Part print with two shaded views. Sizes in mm from the minimum x, y, z corner. A direction names the side the tool comes from. Round coordinates to 2 decimals unless told otherwise and drop trailing zeros. Order: outer loops, then holes, each group sorted by start corner. A loop starts at its lowest first (then second) coordinate and runs counter-clockwise, first axis right, second up. Notation, with made-up numbers: (60.5, -10) - (85.5, -10) arc R14 cw to (85.5, 5) - close; hole circle Ø1 at (-2, -1.75). An arc over 180 degrees is marked (long way). Use one line per item in the form item = value.
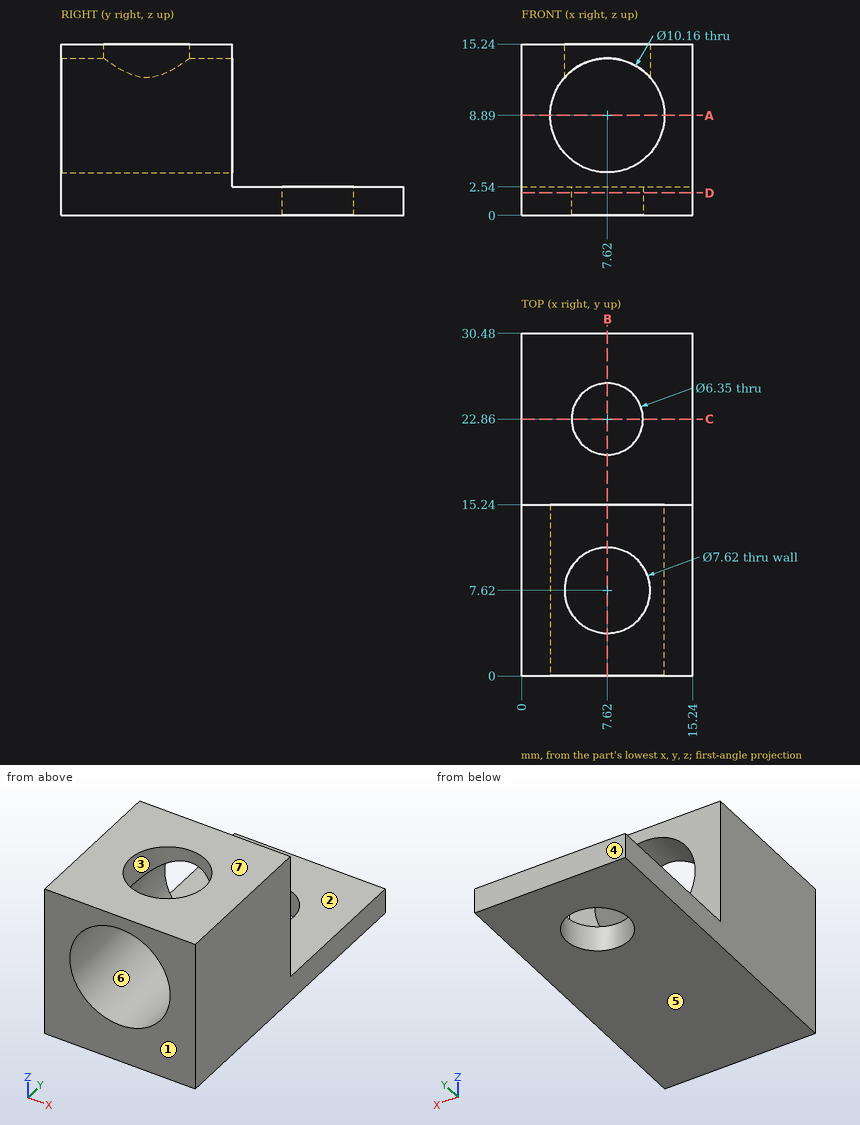
(1) Pull direction Z, two halves, no side cores. Call the marked faces 4, 5, 6 and 7: released by +Z, released by -Z, zero draft, split by the parting line, or undercut.
Report:
face_4 = zero draft
face_5 = released by -Z
face_6 = undercut
face_7 = released by +Z
(2) Slice it at A-A on z = 8.89. Give the cut face in (x, y), then the cut area to 3 significant figures.
Report:
outline = (0, 0) - (2.54, 0) - (2.54, 15.24) - (0, 15.24) - close; (12.7, 0) - (15.24, 0) - (15.24, 15.24) - (12.7, 15.24) - close
area = 77.4 mm2
(3) Slice it at D-D on z = 2. Give the cut face in (x, y) (3 decimals).
Report:
outline = (0, 0) - (15.24, 0) - (15.24, 30.48) - (0, 30.48) - close; hole circle Ø6.35 at (7.62, 22.86)
(4) Probe probe 1 along Y at (x, z) = (7.62, 14); probe 2 along Y at (x, z) = (7.62, 1.05) (3 decimals); probe 3 along Y at (x, z) = (3, 3.75). List the from-to ranges inside material, lowest first. Write a range as [from, to].
Report:
probe_1 = [0, 3.81], [11.43, 15.24]
probe_2 = [0, 19.685], [26.035, 30.48]
probe_3 = [0, 15.24]
(5) Tool access for the marked faces 1, 2 and 3: list every direction of +Z, -Z, +X, -X, +Y, -Y with a clear straight run to the whole face (end or side of a thin tool).
Report:
face_1 = +Z, -Z, +X, -X, -Y
face_2 = +Z, +X, -X, +Y
face_3 = +Z
(6) Slice it at B-B on x = 7.62. Give the cut face in (y, z) (3 decimals), then the cut area to 3 significant figures.
Report:
outline = (0, 0) - (19.685, 0) - (19.685, 2.54) - (15.24, 2.54) - (15.24, 3.81) - (0, 3.81) - close; (0, 13.97) - (3.81, 13.97) - (3.81, 15.24) - (0, 15.24) - close; (11.43, 13.97) - (15.24, 13.97) - (15.24, 15.24) - (11.43, 15.24) - close; (26.035, 0) - (30.48, 0) - (30.48, 2.54) - (26.035, 2.54) - close
area = 90.3 mm2
(7) Pin check, flat tips, straight feed: pin 1 (4 mm diameter, centred on x = 7.62, y = 22.86, fed in from +Z); pin 2 (6 mm diameter, centred on x = 7.62, y = 7.62, fed in from +Z). Stop position of each tip, or through.
Report:
pin_1 = through
pin_2 = 4.79
(8) Slice it at C-C on y = 22.86. Give the cut face in (x, z) (3 decimals).
Report:
outline = (0, 0) - (4.445, 0) - (4.445, 2.54) - (0, 2.54) - close; (10.795, 0) - (15.24, 0) - (15.24, 2.54) - (10.795, 2.54) - close
